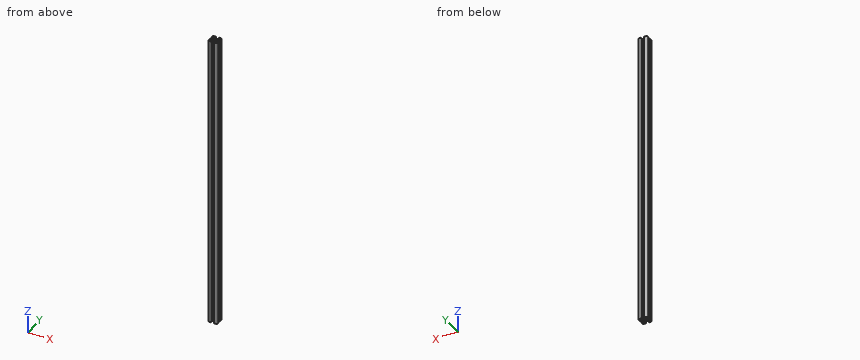
```python
from build123d import *

# Parameters (mm, degrees)
SKETCH_1_R      = 3.4
EXTRUDE_1_DEPTH = 1000


with BuildPart() as part:
    # Эскиз1 → Бобышка-Вытянуть1 (new body)
    with BuildSketch(Plane.XY):
        with BuildLine():
            Line((-15, -8.25), (-15, -12.5))
            ThreePointArc((-15, -12.5), (-14.267766953, -14.267766953), (-12.5, -15))
            Line((-12.5, -15), (-8.25, -15))
            Line((-8.25, -15), (-5.5, -15))
            ThreePointArc((-5.5, -15), (-5.287867966, -14.912132034), (-5.2, -14.7))
            Line((-5.2, -14.7), (-5.2, -14.3))
            ThreePointArc((-5.2, -14.3), (-5.112132034, -14.087867966), (-4.9, -14))
            Line((-4.9, -14), (-4.4, -14))
            ThreePointArc((-4.4, -14), (-4.187867966, -13.912132034), (-4.1, -13.7))
            Line((-4.1, -13.7), (-4.1, -13.3))
            ThreePointArc((-4.1, -13.3), (-4.187867966, -13.087867966), (-4.4, -13))
            Line((-4.4, -13), (-7.95, -13))
            ThreePointArc((-7.95, -13), (-8.162132034, -12.912132034), (-8.25, -12.7))
            Line((-8.25, -12.7), (-8.25, -9.65))
            Line((-8.25, -9.65), (-4, -5.4))
            Line((-4, -5.4), (4, -5.4))
            Line((4, -5.4), (8.25, -9.65))
            Line((8.25, -9.65), (8.25, -12.7))
            ThreePointArc((8.25, -12.7), (8.162132034, -12.912132034), (7.95, -13))
            Line((7.95, -13), (4.4, -13))
            ThreePointArc((4.4, -13), (4.187867966, -13.087867966), (4.1, -13.3))
            Line((4.1, -13.3), (4.1, -13.7))
            ThreePointArc((4.1, -13.7), (4.187867966, -13.912132034), (4.4, -14))
            Line((4.4, -14), (4.9, -14))
            ThreePointArc((4.9, -14), (5.112132034, -14.087867966), (5.2, -14.3))
            Line((5.2, -14.3), (5.2, -14.7))
            ThreePointArc((5.2, -14.7), (5.287867966, -14.912132034), (5.5, -15))
            Line((5.5, -15), (8.25, -15))
            Line((8.25, -15), (12.5, -15))
            ThreePointArc((12.5, -15), (14.267766953, -14.267766953), (15, -12.5))
            Line((15, -12.5), (15, -8.25))
            Line((15, -8.25), (15, -5.5))
            ThreePointArc((15, -5.5), (14.912132034, -5.287867966), (14.7, -5.2))
            Line((14.7, -5.2), (14.3, -5.2))
            ThreePointArc((14.3, -5.2), (14.087867966, -5.112132034), (14, -4.9))
            Line((14, -4.9), (14, -4.4))
            ThreePointArc((14, -4.4), (13.912132034, -4.187867966), (13.7, -4.1))
            Line((13.7, -4.1), (13.3, -4.1))
            ThreePointArc((13.3, -4.1), (13.087867966, -4.187867966), (13, -4.4))
            Line((13, -4.4), (13, -7.95))
            ThreePointArc((13, -7.95), (12.912132034, -8.162132034), (12.7, -8.25))
            Line((12.7, -8.25), (9.65, -8.25))
            Line((9.65, -8.25), (5.4, -4))
            Line((5.4, -4), (5.4, 4))
            Line((5.4, 4), (9.65, 8.25))
            Line((9.65, 8.25), (12.7, 8.25))
            ThreePointArc((12.7, 8.25), (12.912132034, 8.162132034), (13, 7.95))
            Line((13, 7.95), (13, 4.4))
            ThreePointArc((13, 4.4), (13.087867966, 4.187867966), (13.3, 4.1))
            Line((13.3, 4.1), (13.7, 4.1))
            ThreePointArc((13.7, 4.1), (13.912132034, 4.187867966), (14, 4.4))
            Line((14, 4.4), (14, 4.9))
            ThreePointArc((14, 4.9), (14.087867966, 5.112132034), (14.3, 5.2))
            Line((14.3, 5.2), (14.7, 5.2))
            ThreePointArc((14.7, 5.2), (14.912132034, 5.287867966), (15, 5.5))
            Line((15, 5.5), (15, 8.25))
            Line((15, 8.25), (15, 12.5))
            ThreePointArc((15, 12.5), (14.267766953, 14.267766953), (12.5, 15))
            Line((12.5, 15), (8.25, 15))
            Line((8.25, 15), (5.5, 15))
            ThreePointArc((5.5, 15), (5.287867966, 14.912132034), (5.2, 14.7))
            Line((5.2, 14.7), (5.2, 14.3))
            ThreePointArc((5.2, 14.3), (5.112132034, 14.087867966), (4.9, 14))
            Line((4.9, 14), (4.4, 14))
            ThreePointArc((4.4, 14), (4.187867966, 13.912132034), (4.1, 13.7))
            Line((4.1, 13.7), (4.1, 13.3))
            ThreePointArc((4.1, 13.3), (4.187867966, 13.087867966), (4.4, 13))
            Line((4.4, 13), (7.95, 13))
            ThreePointArc((7.95, 13), (8.162132034, 12.912132034), (8.25, 12.7))
            Line((8.25, 12.7), (8.25, 9.65))
            Line((8.25, 9.65), (4, 5.4))
            Line((4, 5.4), (-4, 5.4))
            Line((-4, 5.4), (-8.25, 9.65))
            Line((-8.25, 9.65), (-8.25, 12.7))
            ThreePointArc((-8.25, 12.7), (-8.162132034, 12.912132034), (-7.95, 13))
            Line((-7.95, 13), (-4.4, 13))
            ThreePointArc((-4.4, 13), (-4.187867966, 13.087867966), (-4.1, 13.3))
            Line((-4.1, 13.3), (-4.1, 13.7))
            ThreePointArc((-4.1, 13.7), (-4.187867966, 13.912132034), (-4.4, 14))
            Line((-4.4, 14), (-4.9, 14))
            ThreePointArc((-4.9, 14), (-5.112132034, 14.087867966), (-5.2, 14.3))
            Line((-5.2, 14.3), (-5.2, 14.7))
            ThreePointArc((-5.2, 14.7), (-5.287867966, 14.912132034), (-5.5, 15))
            Line((-5.5, 15), (-8.25, 15))
            Line((-8.25, 15), (-12.5, 15))
            ThreePointArc((-12.5, 15), (-14.267766953, 14.267766953), (-15, 12.5))
            Line((-15, 12.5), (-15, 8.25))
            Line((-15, 8.25), (-15, 5.5))
            ThreePointArc((-15, 5.5), (-14.912132034, 5.287867966), (-14.7, 5.2))
            Line((-14.7, 5.2), (-14.3, 5.2))
            ThreePointArc((-14.3, 5.2), (-14.087867966, 5.112132034), (-14, 4.9))
            Line((-14, 4.9), (-14, 4.4))
            ThreePointArc((-14, 4.4), (-13.912132034, 4.187867966), (-13.7, 4.1))
            Line((-13.7, 4.1), (-13.3, 4.1))
            ThreePointArc((-13.3, 4.1), (-13.087867966, 4.187867966), (-13, 4.4))
            Line((-13, 4.4), (-13, 7.95))
            ThreePointArc((-13, 7.95), (-12.912132034, 8.162132034), (-12.7, 8.25))
            Line((-12.7, 8.25), (-9.65, 8.25))
            Line((-9.65, 8.25), (-5.4, 4))
            Line((-5.4, 4), (-5.4, -4))
            Line((-5.4, -4), (-9.65, -8.25))
            Line((-9.65, -8.25), (-12.7, -8.25))
            ThreePointArc((-12.7, -8.25), (-12.912132034, -8.162132034), (-13, -7.95))
            Line((-13, -7.95), (-13, -4.4))
            ThreePointArc((-13, -4.4), (-13.087867966, -4.187867966), (-13.3, -4.1))
            Line((-13.3, -4.1), (-13.7, -4.1))
            ThreePointArc((-13.7, -4.1), (-13.912132034, -4.187867966), (-14, -4.4))
            Line((-14, -4.4), (-14, -4.9))
            ThreePointArc((-14, -4.9), (-14.087867966, -5.112132034), (-14.3, -5.2))
            Line((-14.3, -5.2), (-14.7, -5.2))
            ThreePointArc((-14.7, -5.2), (-14.912132034, -5.287867966), (-15, -5.5))
            Line((-15, -5.5), (-15, -8.25))
        make_face()
        Circle(SKETCH_1_R, mode=Mode.SUBTRACT)
        with BuildLine():
            Line((-12.45, -9.55), (-10.85, -9.55))
            ThreePointArc((-10.85, -9.55), (-9.930761184, -9.930761184), (-9.55, -10.85))
            Line((-9.55, -10.85), (-9.55, -12.45))
            ThreePointArc((-9.55, -12.45), (-9.930761184, -13.369238816), (-10.85, -13.75))
            Line((-10.85, -13.75), (-12.45, -13.75))
            ThreePointArc((-12.45, -13.75), (-13.369238816, -13.369238816), (-13.75, -12.45))
            Line((-13.75, -12.45), (-13.75, -10.85))
            ThreePointArc((-13.75, -10.85), (-13.369238816, -9.930761184), (-12.45, -9.55))
        make_face(mode=Mode.SUBTRACT)
        with BuildLine():
            Line((-9.55, 12.45), (-9.55, 10.85))
            ThreePointArc((-9.55, 10.85), (-9.930761184, 9.930761184), (-10.85, 9.55))
            Line((-10.85, 9.55), (-12.45, 9.55))
            ThreePointArc((-12.45, 9.55), (-13.369238816, 9.930761184), (-13.75, 10.85))
            Line((-13.75, 10.85), (-13.75, 12.45))
            ThreePointArc((-13.75, 12.45), (-13.369238816, 13.369238816), (-12.45, 13.75))
            Line((-12.45, 13.75), (-10.85, 13.75))
            ThreePointArc((-10.85, 13.75), (-9.930761184, 13.369238816), (-9.55, 12.45))
        make_face(mode=Mode.SUBTRACT)
        with BuildLine():
            Line((12.45, 9.55), (10.85, 9.55))
            ThreePointArc((10.85, 9.55), (9.930761184, 9.930761184), (9.55, 10.85))
            Line((9.55, 10.85), (9.55, 12.45))
            ThreePointArc((9.55, 12.45), (9.930761184, 13.369238816), (10.85, 13.75))
            Line((10.85, 13.75), (12.45, 13.75))
            ThreePointArc((12.45, 13.75), (13.369238816, 13.369238816), (13.75, 12.45))
            Line((13.75, 12.45), (13.75, 10.85))
            ThreePointArc((13.75, 10.85), (13.369238816, 9.930761184), (12.45, 9.55))
        make_face(mode=Mode.SUBTRACT)
        with BuildLine():
            Line((9.55, -12.45), (9.55, -10.85))
            ThreePointArc((9.55, -10.85), (9.930761184, -9.930761184), (10.85, -9.55))
            Line((10.85, -9.55), (12.45, -9.55))
            ThreePointArc((12.45, -9.55), (13.369238816, -9.930761184), (13.75, -10.85))
            Line((13.75, -10.85), (13.75, -12.45))
            ThreePointArc((13.75, -12.45), (13.369238816, -13.369238816), (12.45, -13.75))
            Line((12.45, -13.75), (10.85, -13.75))
            ThreePointArc((10.85, -13.75), (9.930761184, -13.369238816), (9.55, -12.45))
        make_face(mode=Mode.SUBTRACT)
    extrude(amount=EXTRUDE_1_DEPTH)


solid = part.part
```
Source: CAD feature listing. Evaluate the final solid. Frame: model axes, mm. Coordinates: 2 decimals unless noted, no trailing zeros. Answer as a JSON object with one key per item and string values.
Q1. Material intervals for line 1 (X direction, y = 11.75, z = 43.5); line 2 (Y direction, x = -10.5, z = 638), sorted ascending. Write a range as [from, to].
Ans:
{"line 1": "x = [-15, -13.75], [-9.55, -8.25], [8.25, 9.55], [13.75, 15]", "line 2": "y = [-15, -13.7], [-9.6, -8.25], [8.25, 9.6], [13.7, 15]"}
Q2. Section query A-A, the plane z = 608.5. State how many separate pieces and enclosed holes the cut face has, plus the area to 3 significant figures.
Ans:
{"separate pieces": "1", "enclosed holes": "5", "area": "290 mm2"}
Q3. First-contact query: pin 1 Ø6 at (x, z) = (-1.5, 629.5) entering from -Y; pin 2 Ø4 at (x, z) = (-1.5, 401) entering from +Y. Flat tips, straight axial feed; report the tip coordinate or a pass-through.
Ans:
{"pin 1": "stops at y = -14", "pin 2": "stops at y = 5.4"}
